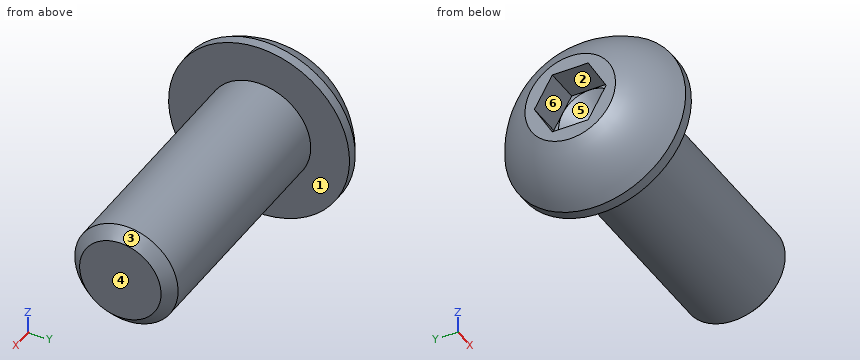
```python
from build123d import *

# Parameters (mm, degrees)
HEX_2_DEPTH = 2.667


with BuildPart() as part:
    # BodySke → BaseBody (revolve)
    with BuildSketch(Plane.XY, mode=Mode.PRIVATE) as basebody_sk:
        with BuildLine():
            Line((23.2664, 0), (23.2664, 3.12928))
            Line((23.2664, 3.12928), (22.42693, 3.96875))
            Line((22.42693, 3.96875), (4.2164, 3.96875))
            Line((4.2164, 3.96875), (4.2164, 6.9469))
            Line((4.2164, 6.9469), (3.429, 6.9469))
            ThreePointArc((3.429, 6.9469), (1.436093175, 5.485019032), (0, 3.47345))
            Line((0, 3.47345), (0, 0))
            Line((0, 0), (23.2664, 0))
        make_face()
    revolve(basebody_sk.sketch.rotate(Axis((0, 0, 0), (1, 0, 0)), 90), axis=Axis((0, 0, 0), (1, 0, 0)))

    # Sketch2 → PreBroach (revolve, cut)
    with BuildSketch(Plane.XY):
        Polygon((0, 2.3876), (2.667, 2.3876), (4.045481503, 0), (0, 0), align=None)
    revolve(axis=Axis((0, 0, 0), (1, 0, 0)), mode=Mode.SUBTRACT)

    # Sketch3 → Hex 2 (cut)
    with BuildSketch(Plane(origin=(0, 0, 0), x_dir=(0, 0, -1), z_dir=(1, 0, 0))):
        Polygon((-2.3876, -1.378481503), (-2.3876, 1.378481503), (0, 2.756963005), (2.3876, 1.378481503), (2.3876, -1.378481503), (0, -2.756963005), align=None)
    extrude(amount=HEX_2_DEPTH, mode=Mode.SUBTRACT)


solid = part.part
```
Source: CAD feature listing. Evaluate the final solid. Frame: model axes, mm. Face numbers are marked on the shaded views. A direction names the side the tool comes from. Give positions to 0.01 mm unless a question says otherwise; leave off trailing zeros. Order: outer loops, then holes, each group sorted by start corner. A loop starts at its lowest first (then second) coordinate and runs counter-clockwise, first axis right, second up. Notation, with made-up numbers: (46.25, 18) -> (105.25, 18) arc R4 ccw to (105.25, 22) -> close; hole circle Ø8 at (22.25, 79.25). An arc over 180 degrees is marked (long way). Use a Markdown table: item, result.
Q1. Pull-direction query (Z, two-part tool) for the marked faces 3, 4, 5 and 6; classes: +Z half, -Z half, draft (parallel to the pull), parting line (faces both ways), or undercut.
A:
| item | result |
|---|---|
| face 3 | parting line |
| face 4 | draft |
| face 5 | undercut |
| face 6 | undercut |
Q2. Section C-C (y = -4.75). Return the cut outline in (x, z), and give its area (3 significant figures).
A:
| item | result |
|---|---|
| outline | (3.43, -5.07) -> (4.22, -5.07) -> (4.22, 5.07) -> (3.43, 5.07) arc R6.2 ccw to start |
| area | 26.7 mm^2 |
Q3. Section B-B (x = 21.5). Return the cut outline in (y, z), and give its area (3 significant figures).
A:
| item | result |
|---|---|
| outline | circle Ø7.94 at (0, 0) |
| area | 49.5 mm^2 |
Q4. Access query for the marked faces 1 and 2. Directions: +Z, -Z, +X, -X, +Y, -Y. A direction counts if a zero-diameter tool reaches every point of the face in a straight line with its end or side. Return the directions, or none.
A:
| item | result |
|---|---|
| face 1 | +X |
| face 2 | -X |
Q5. Material intervals for line 1 (Z direction, x = 10.5, y = -1.75); line 2 (Y direction, x = 10, z = 0.25); line 3 (X direction, y = 0, z = -5), sorted ascending. Write a range as [from, to].
A:
| item | result |
|---|---|
| line 1 | [-3.56, 3.56] |
| line 2 | [-3.96, 3.96] |
| line 3 | [1, 4.22] |
Q6. First-contact query: P1, Ø1, axis at y = 5.5, z = 2.5, coming from the +X side; P2, Ø0.6, axis at y = 1, z = -2, coming from the -X side; P3, Ø5, axis at x = 8, y = 3, coming from the -Z side; P4, Ø1, axis at x = 18.5, z = -5.5, coming from the +Y side. Flat tips, straight axial feed; report the tip coordinate or a pass-through.
A:
| item | result |
|---|---|
| P1 | x = 4.22 |
| P2 | x = 2.67 |
| P3 | z = -3.94 |
| P4 | through |
Q7. Section A-A (y = 5.75). Return the cut outline in (x, z).
A:
| item | result |
|---|---|
| outline | (3.43, -3.9) -> (4.22, -3.9) -> (4.22, 3.9) -> (3.43, 3.9) arc R5.28 ccw to start |
